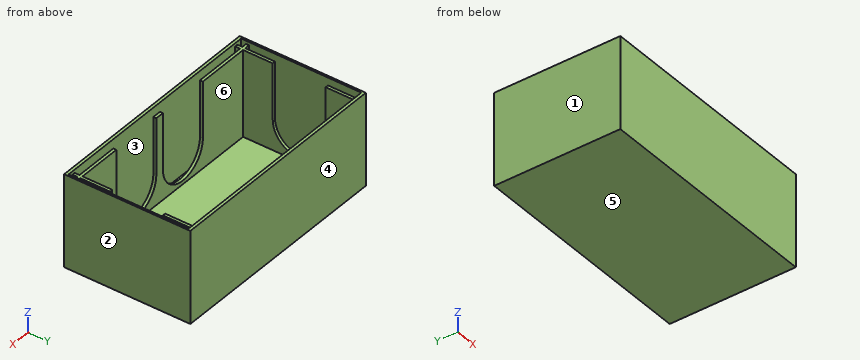
from build123d import *

# Parameters (mm, degrees)
F0_W      = 190
F0_H      = 102.4
F1_DEPTH  = 75
F2_T      = -2.4
F4_DEPTH  = 70
F6_DEPTH  = 2.6
F7_DEPTH  = 176.9
F9_DEPTH  = 2.6
F10_W     = 0.8
F10_H     = 102.4
F11_DEPTH = 75


with BuildPart() as f1:
    # F0 (on Top) → F1 (new body)
    with BuildSketch(Plane.XY):
        with Locations((-3.4108273685, 26.5216542304)):
            Rectangle(F0_W, F0_H)
    extrude(amount=F1_DEPTH)

    # F2
    f2_openings = [f1.faces().sort_by_distance(p)[0] for p in [
        (-3.410827, 26.521654, 75),
    ]]
    offset(amount=F2_T, openings=f2_openings)

    # F3 (on face) → F4 (join)
    with BuildSketch(Plane.XY.offset(2.4)):
        Polygon((-89.6108273685, 75.3216542304), (-92.0108273685, 75.3216542304), (-92.0108273685, -15.8783457696), (-96.0108273685, -15.8783457696), (-96.0108273685, -18.2783457696), (-92.0108273685, -18.2783457696), (-92.0108273685, -22.2783457696), (-89.6108273685, -22.2783457696), (-89.6108273685, -18.2783457696), (82.7891726315, -18.2783457696), (82.7891726315, -22.2783457696), (85.1891726315, -22.2783457696), (85.1891726315, -18.2783457696), (89.1891726315, -18.2783457696), (89.1891726315, -15.8783457696), (85.1891726315, -15.8783457696), (85.1891726315, 75.3216542304), (82.7891726315, 75.3216542304), (82.7891726315, -15.8783457696), (-89.6108273685, -15.8783457696), align=None)
    extrude(amount=F4_DEPTH)

    # F5 (on face) → F6 (cut)
    with BuildSketch(Plane(origin=(82.7891726315, 0, 0), x_dir=(0, -1, 0), z_dir=(-1, 0, 0))):
        with BuildLine():
            Line((-51.2216542304, 72.4), (-51.2216542304, 26.9))
            ThreePointArc((-51.2216542304, 26.9), (-29.7216542304, 5.4), (-8.2216542304, 26.9))
            Line((-8.2216542304, 26.9), (-8.2216542304, 72.4))
            Line((-8.2216542304, 72.4), (-51.2216542304, 72.4))
        make_face()
    extrude(amount=-F6_DEPTH, mode=Mode.SUBTRACT)

    # F5 (on face) → F7 (cut)
    with BuildSketch(Plane(origin=(82.7891726315, 0, 0), x_dir=(0, -1, 0), z_dir=(-1, 0, 0))):
        with BuildLine():
            Line((-51.2216542304, 72.4), (-51.2216542304, 26.9))
            ThreePointArc((-51.2216542304, 26.9), (-29.7216542304, 5.4), (-8.2216542304, 26.9))
            Line((-8.2216542304, 26.9), (-8.2216542304, 72.4))
            Line((-8.2216542304, 72.4), (-51.2216542304, 72.4))
        make_face()
    extrude(amount=F7_DEPTH, mode=Mode.SUBTRACT)

    # F8 (on face) → F9 (cut)
    with BuildSketch(Plane(origin=(0, -15.8783457696, 0), x_dir=(-1, 0, 0), z_dir=(0, 1, 0))):
        with BuildLine():
            Line((3.5, 72.4), (3.5, 26.9))
            ThreePointArc((3.5, 26.9), (25, 5.4), (46.5, 26.9))
            Line((46.5, 26.9), (46.5, 72.4))
            Line((46.5, 72.4), (3.5, 72.4))
        make_face()
        with BuildLine():
            Line((-46.5, 72.4), (-46.5, 26.9))
            ThreePointArc((-46.5, 26.9), (-25, 5.4), (-3.5, 26.9))
            Line((-3.5, 26.9), (-3.5, 72.4))
            Line((-3.5, 72.4), (-46.5, 72.4))
        make_face()
    extrude(amount=-F9_DEPTH, mode=Mode.SUBTRACT)

    # F10 (on face) → F11 (cut)
    with BuildSketch(Plane.XY.offset(75)):
        with Locations((-98.0108273685, 26.5216542304)):
            Rectangle(F10_W, F10_H)
        with Locations((91.1891726315, 26.5216542304)):
            Rectangle(F10_W, F10_H)
    extrude(amount=-F11_DEPTH, mode=Mode.SUBTRACT)


solid = f1.part
The model under review builds one solid part; all positions refer to its coordinate system, in mm. Face numbers are marked on the shaded views. A direction names the side the tool comes from. Coordinates: 2 decimals unless noted, no trailing zeros. Loops run counter-clockwise (first coordinate to the right, second up) from the corner with the lowest first, then second, coordinate; pieces in that order, holes last.
(1) Consider section C-C, the plane x = 48.5. Give the boundary of the cut face in (y, z), plus the area to 3 significant figures.
Determined:
outline: (-24.68, 0) - (77.72, 0) - (77.72, 75) - (75.32, 75) - (75.32, 2.4) - (-15.88, 2.4) - (-15.88, 72.4) - (-18.28, 72.4) - (-18.28, 2.4) - (-22.28, 2.4) - (-22.28, 75) - (-24.68, 75) - close
area: 762 mm2
(2) Tool access review of the marked faces 5 and 6: name each direction out of +Z, -Z, +X, -X, +Y, -Y from which nothing blocks a thin tool from reaching the whole face with its end or side.
Determined:
face 5: -Z, +X, -X, +Y, -Y
face 6: +Z
(3) Consider section B-B, the plane z = 57.5. Give the number of separate pieces and of enclosed holes in the cut face, plus the area to 3 significant figures.
Determined:
separate pieces: 2
enclosed holes: 3
area: 1,710 mm2
(4) Insertion check: P1, Ø1.5, axis at x = -3.5, y = 59.5, coming from the +Z side. The pin has a flat end and moves straight along its axis. Give the tip position at first contact, or say it passes through.
Determined:
P1: stops at z = 2.4
(5) Wall thickness on L1, parallel to X at y = 1, z = 58; L2, parallel to Y at x = -3, z = 32; L3, parallel to Y at x = 33.5, z = 16.5: over which ranges is each line inside the solid? List them lowest first.
Determined:
L1: x = -97.61 to -96.01, -92.01 to -89.61, 82.79 to 85.19, 89.19 to 90.79
L2: y = -24.68 to -22.28, -18.28 to -15.88, 75.32 to 77.72
L3: y = -24.68 to -22.28, 75.32 to 77.72
(6) Consider section A-A, the plane y = 2. Give the boundary of the cut face in (x, z).
Determined:
outline: (-97.61, 0) - (90.79, 0) - (90.79, 75) - (89.19, 75) - (89.19, 2.4) - (85.19, 2.4) - (85.19, 72.4) - (82.79, 72.4) - (82.79, 2.4) - (-89.61, 2.4) - (-89.61, 72.4) - (-92.01, 72.4) - (-92.01, 2.4) - (-96.01, 2.4) - (-96.01, 75) - (-97.61, 75) - close
(7) Consider section D-D, the plane x = -25. Give the boundary of the cut face in (y, z), plus the area to 3 significant figures.
Determined:
outline: (-24.68, 0) - (77.72, 0) - (77.72, 75) - (75.32, 75) - (75.32, 2.4) - (-15.88, 2.4) - (-15.88, 5.4) - (-18.28, 5.4) - (-18.28, 2.4) - (-22.28, 2.4) - (-22.28, 75) - (-24.68, 75) - close
area: 601 mm2
(8) Draft analysis for pull direction X (two halves, no side actions). For the marked faces 1, 2, 3 and 4, state which applies: +X half, -X half, draft (parallel to the pull), parting line (faces both ways), or undercut.
Determined:
face 1: -X half
face 2: +X half
face 3: undercut
face 4: draft
